For this review, use the dimensioned drawing (mm, ordinates from the lowest corner) and the shaded views. Coordinates: 2 decimals unless noted, no trailing zeros. Loops run counter-clockwise (first coordinate to the right, second up) from the corner with the lowest first, then second, coordinate; pieces in that order, holes last. Notation, with made-up numbers: M 63.25,32 L 103.25,32 A24 cw 103.25,46 Z; hole C 33.5,-1 d4. An arc over 180 degrees is marked long. Use CSV: the item, a comma, the result in double quotes. Start each with the question number.
1. Add section C-C, the plane z = 3.25. Write out the cut boundary in (x, y), then the cut area to 3 significant figures.
2. For L1, parallel to Y at x = 38.1, z = 5; L2, parallel to Y at x = 36, z = 1.5; L3, parallel to X at y = 67.01, z = 3.25, list the stretches that pass through material, from the lowest coordinate up.
3. Add section A-A, the plane y = 183.69. Write out the cut boundary in (x, z), then the cut area to 3 significant figures.
4. Add section D-D, the plane y = 15. Write out the cut boundary in (x, z), then the cut area to 3 significant figures.
5. Add section B-B, the plane x = 50.5. Write out the cut boundary in (y, z), then the cut area to 3 significant figures.
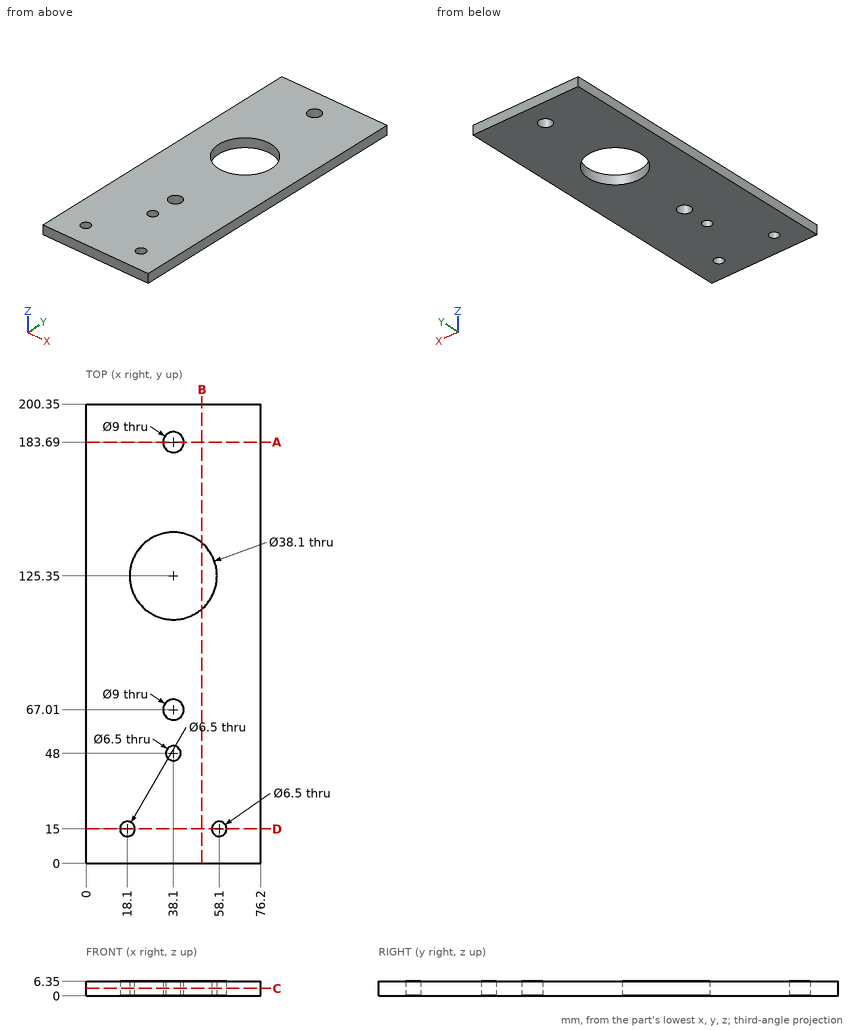
Computed:
1,outline,"M 0,0 L 76.2,0 L 76.2,200.35 L 0,200.35 Z; hole C 18.1,15 d6.5; hole C 38.1,125.35 d38.1; hole C 38.1,67.01 d9; hole C 38.1,183.69 d9; hole C 38.1,48 d6.5; hole C 58.1,15 d6.5"
1,area,"13,900 mm^2"
2,L1,"y = 0 to 44.75, 51.25 to 62.51, 71.51 to 106.3, 144.4 to 179.19, 188.19 to 200.35"
2,L2,"y = 0 to 45.52, 50.48 to 63.03, 70.99 to 106.42, 144.28 to 179.71, 187.67 to 200.35"
2,L3,"x = 0 to 33.6, 42.6 to 76.2"
3,outline,"M 0,0 L 33.6,0 L 33.6,6.35 L 0,6.35 Z; M 42.6,0 L 76.2,0 L 76.2,6.35 L 42.6,6.35 Z"
3,area,"427 mm^2"
4,outline,"M 0,0 L 14.85,0 L 14.85,6.35 L 0,6.35 Z; M 21.35,0 L 54.85,0 L 54.85,6.35 L 21.35,6.35 Z; M 61.35,0 L 76.2,0 L 76.2,6.35 L 61.35,6.35 Z"
4,area,"401 mm^2"
5,outline,"M 0,0 L 110.89,0 L 110.89,6.35 L 0,6.35 Z; M 139.81,0 L 200.35,0 L 200.35,6.35 L 139.81,6.35 Z"
5,area,"1,090 mm^2"
